```python
from build123d import *

# Parameters (mm, degrees)
EXTRUDE_1_DEPTH     = 2.6
FILLET_1_R          = 2
SKETCH_2_W          = 2.6
SKETCH_2_H          = 2.6
SKETCH_2_R          = 0.6
EXTRUDE_2_DEPTH     = 2
SKETCH_4_W          = 2.6
SKETCH_4_H          = 1
SKETCH_4_H_2        = 0.5
CUT_EXTRUDE_1_DEPTH = 12.340634903


with BuildPart() as part:
    # 草图1 → 凸台-拉伸1 (new body)
    with BuildSketch(Plane.XY):
        Polygon((6.6, 6.1), (-6.6, 6.1), (-6.6, -6.1), (-5, -6.1), (-5, 5.1), (5, 5.1), (5, -6.1), (6.6, -6.1), align=None)
    extrude(amount=EXTRUDE_1_DEPTH)

    # 圆角1
    fillet_1_edges = [part.edges().sort_by_distance(p)[0] for p in [
        (5, 5.1, 1.3),
        (-5, 5.1, 1.3),
        (-6.6, 6.1, 1.3),
        (6.6, 6.1, 1.3),
    ]]
    fillet(fillet_1_edges, radius=FILLET_1_R)

    # 草图2 → 凸台-拉伸2 (add)
    # profile 1 of 2: a face of its own
    with BuildSketch(Plane.XZ.offset(6.1)):
        with Locations((-7.9, 1.3)):
            Rectangle(SKETCH_2_W, SKETCH_2_H)
        with Locations(Location((-7.9, 1.3, 0), (0, 0, 270))):
            Circle(SKETCH_2_R, mode=Mode.SUBTRACT)
    # profile 2 of 2: a face of its own
    with BuildSketch(Plane.XZ.offset(6.1)):
        with Locations((7.9, 1.3)):
            Rectangle(SKETCH_2_W, SKETCH_2_H)
        with Locations(Location((7.9, 1.3, 0), (0, 0, 270))):
            Circle(SKETCH_2_R, mode=Mode.SUBTRACT)
    extrude(amount=-EXTRUDE_2_DEPTH)

    # 草图4 → 切除-拉伸1 (cut, through all)
    with BuildSketch(Plane.XY.offset(2.6)):
        with Locations((-7.9, -5.6)):
            Rectangle(SKETCH_4_W, SKETCH_4_H)
        with Locations((7.9, -4.35)):
            Rectangle(SKETCH_4_W, SKETCH_4_H_2)
    extrude(amount=-CUT_EXTRUDE_1_DEPTH, mode=Mode.SUBTRACT)


solid = part.part
```
Build history of the part. All positions in model axes, mm. A direction names the side the tool comes from. Round coordinates to 2 decimals unless told otherwise and drop trailing zeros. Write each loop counter-clockwise with the first axis right and the second up, starting at its lowest first coordinate (ties: lowest second). Pieces come first, ordered by that corner, then holes. Notation, with made-up numbers: (-34, 51) -> (0, 51) arc R21 ccw to (0, 67) -> close; hole circle Ø9 at (40, 44.25). An arc over 180 degrees is marked (long way). Put each result on its own line as item: value.
Item 1: Flat gauge pins, fed straight in: P1, Ø1.5, axis at x = 0.5, z = 2, coming from the -Y side; P2, Ø0.8, axis at y = -1.5, z = 1.5, coming from the +X side; P3, Ø0.8, axis at y = -1.5, z = 1, coming from the -X side. Where does each tip first touch, or does it go through?
Here are the results:
P1: stops at y = 5.1
P2: stops at x = 6.6
P3: stops at x = -6.6
Item 2: Slice it at A-A, the plane y = 2.75. Give the cut face in (x, z), plus the area to 3 significant figures.
Here are the results:
outline: (-6.6, 0) -> (-5, 0) -> (-5, 2.6) -> (-6.6, 2.6) -> close; (5, 0) -> (6.6, 0) -> (6.6, 2.6) -> (5, 2.6) -> close
area: 8.32 mm^2
Item 3: Slice it at D-D, the plane z = 2.35. Give the cut face in (x, y).
Here are the results:
outline: (-9.2, -5.1) -> (-6.6, -5.1) -> (-6.6, -6.1) -> (-5, -6.1) -> (-5, 3.1) arc R2 cw to (-3, 5.1) -> (3, 5.1) arc R2 cw to (5, 3.1) -> (5, -6.1) -> (9.2, -6.1) -> (9.2, -4.6) -> (6.6, -4.6) -> (6.6, 4.1) arc R2 ccw to (4.6, 6.1) -> (-4.6, 6.1) arc R2 ccw to (-6.6, 4.1) -> (-6.6, -4.1) -> (-9.2, -4.1) -> close
Item 4: Tool access for faces 1 (the face through (6.6, 0, 1)), 2 (the face through (-7, -5.1, 1)), 3 (the face through (0, 5.1, 1)), 4 (the face through (9.2, -5, 1)), 5 (the face through (-6.6, 0, 1)): list every direction of +Z, -Z, +X, -X, +Y, -Y with a clear straight run to the whole face (end or side of a thin tool).
Here are the results:
face 1: +Z, -Z, +X, +Y
face 2: +Z, -Z, -X, -Y
face 3: +Z, -Z, -Y
face 4: +Z, -Z, +X, +Y, -Y
face 5: +Z, -Z, -X, +Y
Item 5: Slice it at B-B, the plane z = 1.3. Give the cut face in (x, y).
Here are the results:
outline: (-9.2, -5.1) -> (-8.5, -5.1) -> (-8.5, -4.1) -> (-9.2, -4.1) -> close; (-7.3, -5.1) -> (-6.6, -5.1) -> (-6.6, -6.1) -> (-5, -6.1) -> (-5, 3.1) arc R2 cw to (-3, 5.1) -> (3, 5.1) arc R2 cw to (5, 3.1) -> (5, -6.1) -> (7.3, -6.1) -> (7.3, -4.6) -> (6.6, -4.6) -> (6.6, 4.1) arc R2 ccw to (4.6, 6.1) -> (-4.6, 6.1) arc R2 ccw to (-6.6, 4.1) -> (-6.6, -4.1) -> (-7.3, -4.1) -> close; (8.5, -6.1) -> (9.2, -6.1) -> (9.2, -4.6) -> (8.5, -4.6) -> close
Item 6: Slice it at C-C, the plane x = -7.9. Give the cut face in (y, z).
Here are the results:
outline: (-5.1, 0) -> (-4.1, 0) -> (-4.1, 0.7) -> (-5.1, 0.7) -> close; (-5.1, 1.9) -> (-4.1, 1.9) -> (-4.1, 2.6) -> (-5.1, 2.6) -> close
Item 7: Two-plate mould, pull along X, no slides. Class faces 6 (the face through (-4.43, 4.5, 1.32)), 7 (the face through (-6, -6.1, 1)), 8 (the face through (-6, 5.53, 1.32)), 9 (the face through (-8.265, -4.607, 1.776)): pulls with the +X half, pulls with the -X half, needs draft (parallel to the pull), parting line crosses it, or undercut.
Here are the results:
face 6: undercut
face 7: needs draft
face 8: pulls with the -X half
face 9: undercut
Item 8: Wall check: probe 1 along X at (y, z) = (-5.2, 1.3); probe 2 along X at (y, z) = (-4.75, 1.3); probe 3 along X at (y, z) = (0.25, 2.55). Give the ranges that are in metal, low to high. Write a range as from..to.
Here are the results:
probe 1: x = -6.6..-5, 5..7.3, 8.5..9.2
probe 2: x = -9.2..-8.5, -7.3..-5, 5..7.3, 8.5..9.2
probe 3: x = -6.6..-5, 5..6.6
